Study the drawing (mm; zero at the part's minimum x, y, z) and answer. Coordinates: 2 decimals unless noted, no trailing zeros. Order: outer loops, then holes, each group sorted by start corner. A loop starts at its lowest first (then second) coordinate and runs counter-clockwise, first axis right, second up. Notation, with made-up numbers: (-18.75, -12) -> (8.25, -12) arc R14 ccw to (8.25, -7) -> close; hole circle Ø1 at (22, -19). An arc over 180 degrees is marked (long way). One line per question, with ' | ' between items.
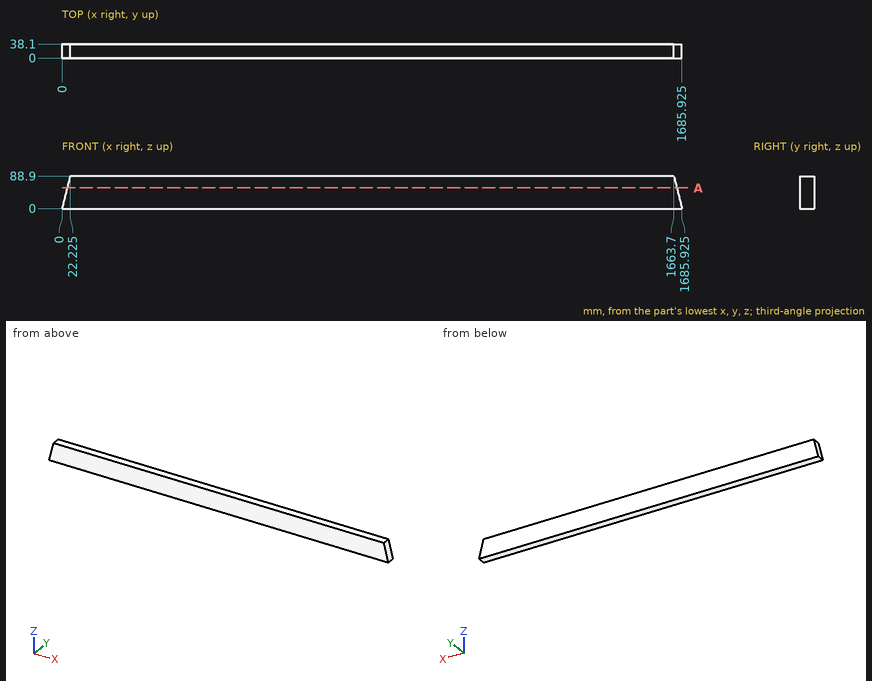
Item 1: Section A-A, the plane z = 56.5 is taken. Give the vertices of the cut face in (x, y) (3 decimals).
Computed values:
outline: (14.125, 0) -> (1671.8, 0) -> (1671.8, 38.1) -> (14.125, 38.1) -> close
Item 2: Each of these flat-tipped pins is pushed along its axis until it touches: pin 1 Ø1.5 at (x, y) = (815.5, 12) entering from -Z; pin 2 Ø5 at (y, z) = (21, 54) entering from +X; pin 3 Ø1.5 at (y, z) = (11.5, 74.5) entering from +X; pin 4 Ø12 at (y, z) = (28.5, 23) entering from -X. Where does it stop, or does it pass through?
Computed values:
pin 1: stops at z = 0 | pin 2: stops at x = 1673.05 | pin 3: stops at x = 1667.49 | pin 4: stops at x = 4.25
Item 3: Find the intervals of material crossed by L1, parallel to X at y = 28, z = 77.5 (3 decimals); L2, parallel to X at y = 32, z = 72.5 (3 decimals), in increasing order.
Computed values:
L1: x = 19.375 to 1666.55 | L2: x = 18.125 to 1667.8
